from build123d import *

# Parameters (mm, degrees)
F0_W     = 96.270095
F0_H     = 50.328871
F1_DEPTH = 50.8
F2_W     = 96.270095
F2_H     = 17.292487
F3_DEPTH = 11.43
F4_W     = 44.908839
F4_H     = 17.292487
F5_DEPTH = 70.104


with BuildPart() as f1:
    # F0 (on Top) → F1 (new body)
    with BuildSketch(Plane.XY):
        with Locations((6.065273, -2.710015)):
            Rectangle(F0_W, F0_H)
    extrude(amount=F1_DEPTH)

    # F2 (on face) → F3 (cut)
    with BuildSketch(Plane.XZ.offset(27.874451)):
        with Locations((6.065273, 26.432386)):
            Rectangle(F2_W, F2_H)
    extrude(amount=-F3_DEPTH, mode=Mode.SUBTRACT)

    # F4 (on face) → F5 (cut)
    with BuildSketch(Plane.XZ.offset(16.444451)):
        with Locations((5.678129, 26.432386)):
            Rectangle(F4_W, F4_H)
    extrude(amount=-F5_DEPTH, mode=Mode.SUBTRACT)


solid = f1.part
Input: part model. Units: mm. Frame: model coordinates. A direction names the side the tool comes from. Coordinates: 2 decimals unless noted, no trailing zeros. Loops run counter-clockwise (first coordinate to the right, second up) from the corner with the lowest first, then second, coordinate; pieces in that order, holes last.
Q1. Material intervals for line 1 (Z direction, x = -6, y = -3); line 2 (X direction, y = 2, z = 26); line 3 (Y direction, x = 32.5, z = 23), sorted ascending.
Q2. Cut plane C-C (y = 1). Output: boundary loops of the cut face in (x, z).
Q3. Draft query along Z for faces 1 (the face through (5, -2, 50.8)), 2 (the face through (-16.776, 3, 26)), 3 (the face through (54.2, -3, 25)), 4 (the face through (5, -9, 35.079)). Return one class per face: +Z half, -Z half, draft (parallel to the pull), parting line (faces both ways), or undercut.
Q4. Set-up query: faces 5 (the face through (5, -9, 17.786)), 6 (the face through (5, -2, 0)), 7 (the face through (41, -16.444, 27)), 8 (the face through (28.133, 3, 26)). Return all of +Z, -Z, +X, -X, +Y, -Y with unobstructed straight access to the full face (end or side cutting, diameter ignored); none if empty.
Q5. Cut plane D-D (x = 46.5). Output: boundary loops of the cut face in (y, z).
Q6. Cut plane B-B (z = 27.5). Output: boundary loops of the cut face in (x, y), then the cut area to 3 significant figures.
Q7. Contact query for flat-ended pins moving along their axis: pin 1 (5 mm diameter, centred on x = -34.5, z = 25.5, fed in from -Y); pin 2 (5 mm diameter, centred on x = 35, y = 3, fed in from -Z). Output: stop coordinate, or through.
Q8. Cut plane A-A (x = -15.5). Output: boundary loops of the cut face in (y, z), then the cut area to 3 significant figures.
Working result:
1. line 1: z = 0 to 17.79, 35.08 to 50.8
1. line 2: x = -42.07 to -16.78, 28.13 to 54.2
1. line 3: y = -16.44 to 22.45
2. outline: (-42.07, 0) - (54.2, 0) - (54.2, 50.8) - (-42.07, 50.8) - close; hole (-16.78, 17.79) - (28.13, 17.79) - (28.13, 35.08) - (-16.78, 35.08) - close
3. face 1: +Z half
3. face 2: undercut
3. face 3: draft
3. face 4: undercut
4. face 5: -Y
4. face 6: -Z, +X, -X, +Y, -Y
4. face 7: +X, -X, -Y
4. face 8: +Y, -Y
5. outline: (-27.87, 0) - (22.45, 0) - (22.45, 50.8) - (-27.87, 50.8) - (-27.87, 35.08) - (-16.44, 35.08) - (-16.44, 17.79) - (-27.87, 17.79) - close
6. outline: (-42.07, -16.44) - (-16.78, -16.44) - (-16.78, 22.45) - (-42.07, 22.45) - close; (28.13, -16.44) - (54.2, -16.44) - (54.2, 22.45) - (28.13, 22.45) - close
6. area: 2,000 mm2
7. pin 1: stops at y = -16.44
7. pin 2: stops at z = 0
8. outline: (-27.87, 0) - (22.45, 0) - (22.45, 17.79) - (-27.87, 17.79) - close; (-27.87, 35.08) - (22.45, 35.08) - (22.45, 50.8) - (-27.87, 50.8) - close
8. area: 1,690 mm2
